from build123d import *

# Parameters (mm, degrees)
SKETCH_1_W          = 30
SKETCH_1_H          = 30
EXTRUDE_1_DEPTH     = 65
CUT_EXTRUDE_1_DEPTH = 54
CUT_EXTRUDE_2_DEPTH = 25
EXTRUDE_START       = -5.5
EXTRUDE_2_DEPTH     = 49.5
FILLET_1_R          = 0.1
SKETCH_6_R          = 3.5
CUT_EXTRUDE_3_DEPTH = 5
EXTRUDE_START_2     = 0.2
SKETCH_7_R          = 4.5
SKETCH_7_R_2        = 3.5
EXTRUDE_3_DEPTH     = 0.2
SKETCH_8_R          = 2.1
EXTRUDE_4_DEPTH     = 8
SKETCH_9_R          = 0.3
CUT_EXTRUDE_4_DEPTH = 8
CHAMFER_1_SIZE      = 1
CHAMFER_1_SIZE2     = 0.577350269
FILLET_2_R          = 0.1
FILLET_3_R          = 0.2
SKETCH_10_R         = 1.25
CUT_EXTRUDE_5_DEPTH = 5
SKETCH_11_R         = 1.25
CUT_EXTRUDE_6_DEPTH = 5
CUT_EXTRUDE_START   = -5
SKETCH_12_R         = 1.25
CUT_EXTRUDE_7_DEPTH = 5


with BuildPart() as part:
    # 草图1 → 凸台-拉伸1 (new body)
    with BuildSketch(Plane.XY):
        with Locations((0, 15)):
            Rectangle(SKETCH_1_W, SKETCH_1_H)
    extrude(amount=-EXTRUDE_1_DEPTH)

    # 草图2 → 切除-拉伸1 (cut)
    with BuildSketch(Plane(origin=(0, 0, -65), x_dir=(-1, 0, 0), z_dir=(0, 0, -1))):
        with BuildLine():
            Line((-9, 0.677124344), (-9, 0))
            Line((-9, 0), (-6, 0))
            Line((-6, 0), (-6, 0.677124344))
            ThreePointArc((-6, 0.677124344), (-5.719957697, 1.088161527), (-5.55, 1.555590279))
            Line((-5.55, 1.555590279), (-5.55, 2.8))
            Line((-5.55, 2.8), (-9.45, 2.8))
            Line((-9.45, 2.8), (-9.45, 1.555590279))
            ThreePointArc((-9.45, 1.555590279), (-9.280042303, 1.088161527), (-9, 0.677124344))
        make_face()
        with BuildLine():
            Line((5.55, 2.8), (5.55, 1.555590279))
            ThreePointArc((5.55, 1.555590279), (5.719957697, 1.088161527), (6, 0.677124344))
            Line((6, 0.677124344), (6, 0))
            Line((6, 0), (9, 0))
            Line((9, 0), (9, 0.677124344))
            ThreePointArc((9, 0.677124344), (9.280042303, 1.088161527), (9.45, 1.555590279))
            Line((9.45, 1.555590279), (9.45, 2.8))
            Line((9.45, 2.8), (5.55, 2.8))
        make_face()
    extrude(amount=-CUT_EXTRUDE_1_DEPTH, mode=Mode.SUBTRACT)

    # 草图3 → 切除-拉伸2 (cut)
    with BuildSketch(Plane(origin=(0, 0, -65), x_dir=(-1, 0, 0), z_dir=(0, 0, -1))):
        with BuildLine():
            Line((-14.322875656, 9), (-15, 9))
            Line((-15, 9), (-15, 6))
            Line((-15, 6), (-14.322875656, 6))
            ThreePointArc((-14.322875656, 6), (-13.911838473, 5.719957697), (-13.444409721, 5.55))
            Line((-13.444409721, 5.55), (-12.2, 5.55))
            Line((-12.2, 5.55), (-12.2, 9.45))
            Line((-12.2, 9.45), (-13.444409721, 9.45))
            ThreePointArc((-13.444409721, 9.45), (-13.911838473, 9.280042303), (-14.322875656, 9))
        make_face()
        with BuildLine():
            Line((-12.2, 20.55), (-13.444409721, 20.55))
            ThreePointArc((-13.444409721, 20.55), (-13.911838473, 20.719957697), (-14.322875656, 21))
            Line((-14.322875656, 21), (-15, 21))
            Line((-15, 21), (-15, 24))
            Line((-15, 24), (-14.322875656, 24))
            ThreePointArc((-14.322875656, 24), (-13.911838473, 24.280042303), (-13.444409721, 24.45))
            Line((-13.444409721, 24.45), (-12.2, 24.45))
            Line((-12.2, 24.45), (-12.2, 20.55))
        make_face()
        with BuildLine():
            Line((14.322875656, 21), (15, 21))
            Line((15, 21), (15, 24))
            Line((15, 24), (14.322875656, 24))
            ThreePointArc((14.322875656, 24), (13.911838473, 24.280042303), (13.444409721, 24.45))
            Line((13.444409721, 24.45), (12.2, 24.45))
            Line((12.2, 24.45), (12.2, 20.55))
            Line((12.2, 20.55), (13.444409721, 20.55))
            ThreePointArc((13.444409721, 20.55), (13.911838473, 20.719957697), (14.322875656, 21))
        make_face()
        with BuildLine():
            Line((12.2, 9.45), (13.444409721, 9.45))
            ThreePointArc((13.444409721, 9.45), (13.911838473, 9.280042303), (14.322875656, 9))
            Line((14.322875656, 9), (15, 9))
            Line((15, 9), (15, 6))
            Line((15, 6), (14.322875656, 6))
            ThreePointArc((14.322875656, 6), (13.911838473, 5.719957697), (13.444409721, 5.55))
            Line((13.444409721, 5.55), (12.2, 5.55))
            Line((12.2, 5.55), (12.2, 9.45))
        make_face()
    extrude(amount=-CUT_EXTRUDE_2_DEPTH, mode=Mode.SUBTRACT)

    # 草图5 → 凸台-拉伸2 (add)
    with BuildSketch(Plane(origin=(0, 0, -65), x_dir=(-1, 0, 0), z_dir=(0, 0, -1)).offset(EXTRUDE_START)):
        with BuildLine():
            Line((-1.5, 30.677124344), (-1.5, 30))
            Line((-1.5, 30), (-0.5, 30))
            Line((-0.5, 30), (-0.5, 31.07225346))
            Line((-0.5, 31.07225346), (-1.165769145, 32.5))
            Line((-1.165769145, 32.5), (-1.95, 32.5))
            Line((-1.95, 32.5), (-1.95, 31.555590279))
            ThreePointArc((-1.95, 31.555590279), (-1.780042303, 31.088161527), (-1.5, 30.677124344))
        make_face()
        with BuildLine():
            Line((1.5, 30), (1.5, 30.677124344))
            ThreePointArc((1.5, 30.677124344), (1.780042303, 31.088161527), (1.95, 31.555590279))
            Line((1.95, 31.555590279), (1.95, 32.5))
            Line((1.95, 32.5), (1.165769145, 32.5))
            Line((1.165769145, 32.5), (0.5, 31.07225346))
            Line((0.5, 31.07225346), (0.5, 30))
            Line((0.5, 30), (1.5, 30))
        make_face()
    extrude(amount=-EXTRUDE_2_DEPTH)

    # 圆角1
    fillet_1_edges = [part.edges().sort_by_distance(p)[0] for p in [
        (1.557884573, 32.5, -10),
        (1.95, 32.5, -34.75),
        (1.165769145, 32.5, -34.75),
        (1.557884573, 32.5, -59.5),
        (-1.557884573, 32.5, -10),
        (-1.165769145, 32.5, -34.75),
        (-1.95, 32.5, -34.75),
        (-1.557884573, 32.5, -59.5),
    ]]
    fillet(fillet_1_edges, radius=FILLET_1_R)

    # 草图6 → 切除-拉伸3 (cut)
    with BuildSketch(Plane.XY):
        with Locations((0, 15)):
            Circle(SKETCH_6_R)
    extrude(amount=-CUT_EXTRUDE_3_DEPTH, mode=Mode.SUBTRACT)

    # 草图7 → 凸台-拉伸3 (add)
    with BuildSketch(Plane.XY.offset(EXTRUDE_START_2)):
        with Locations(Location((0, 15, 0), (0, 0, 180))):
            Circle(SKETCH_7_R)
        with Locations((0, 15)):
            Circle(SKETCH_7_R_2, mode=Mode.SUBTRACT)
    extrude(amount=-EXTRUDE_3_DEPTH)

    # 草图8 → 凸台-拉伸4 (add)
    with BuildSketch(Plane.XY.offset(-5)):
        with Locations((0, 15)):
            Circle(SKETCH_8_R)
    extrude(amount=EXTRUDE_4_DEPTH)

    # 草图9 → 切除-拉伸4 (cut)
    with BuildSketch(Plane.XY.offset(3)):
        with Locations((0, 15)):
            Circle(SKETCH_9_R)
    extrude(amount=-CUT_EXTRUDE_4_DEPTH, mode=Mode.SUBTRACT)

    # 倒角1
    chamfer_1_edges = [part.edges().sort_by_distance(p)[0] for p in [
        (-2.1, 15, 3),
    ]]
    chamfer_1_side = [part.faces().sort_by_distance(p)[0] for p in [
        (-2.1, 15, -1),
    ]]
    chamfer(chamfer_1_edges, length=CHAMFER_1_SIZE, length2=CHAMFER_1_SIZE2, reference=chamfer_1_side[0])

    # 圆角2
    fillet_2_edges = [part.edges().sort_by_distance(p)[0] for p in [
        (-1.522649731, 15, 3),
    ]]
    fillet(fillet_2_edges, radius=FILLET_2_R)

    # 圆角3
    fillet_3_edges = [part.edges().sort_by_distance(p)[0] for p in [
        (15, 3, -65),
        (-15, 15, -65),
        (-15, 22.5, -40),
        (-15, 24, -52.5),
        (-15, 21, -52.5),
        (-15, 3, -65),
        (0, 30, -65),
        (-15, 7.5, -40),
        (-15, 9, -52.5),
        (-15, 6, -52.5),
        (12, 0, -65),
        (7.5, 0, -11),
        (6, 0, -38),
        (9, 0, -38),
        (0, 0, -65),
        (-15, 27, -65),
        (-7.5, 0, -11),
        (-9, 0, -38),
        (-6, 0, -38),
        (0, 30, 0),
        (15, 15, 0),
        (0, 0, 0),
        (-15, 15, 0),
        (15, 15, -65),
        (-12, 0, -65),
        (15, 7.5, -40),
        (15, 6, -52.5),
        (15, 9, -52.5),
        (-15, 30, -32.5),
        (15, 30, -32.5),
        (15, 0, -32.5),
        (-15, 0, -32.5),
        (15, 27, -65),
        (15, 22.5, -40),
        (15, 21, -52.5),
        (15, 24, -52.5),
    ]]
    fillet(fillet_3_edges, radius=FILLET_3_R)

    # 草图10 → 切除-拉伸5 (cut)
    with BuildSketch(Plane.XY):
        with Locations((-12.25, 3.75)):
            Circle(SKETCH_10_R)
        with Locations((12.25, 3.75)):
            Circle(SKETCH_10_R)
    extrude(amount=-CUT_EXTRUDE_5_DEPTH, mode=Mode.SUBTRACT)

    # 草图11 → 切除-拉伸6 (cut)
    with BuildSketch(Plane(origin=(15, 0, 0), x_dir=(0, 0, -1), z_dir=(1, 0, 0))):
        with Locations((3.75, 3.75)):
            Circle(SKETCH_11_R)
    extrude(amount=-CUT_EXTRUDE_6_DEPTH, mode=Mode.SUBTRACT)

    # 草图12 → 切除-拉伸7 (cut)
    with BuildSketch(Plane.ZY.offset(15).offset(CUT_EXTRUDE_START)):
        with Locations(Location((-3.75, 3.75, 0), (0, 0, 180))):
            Circle(SKETCH_12_R)
    extrude(amount=CUT_EXTRUDE_7_DEPTH, mode=Mode.SUBTRACT)


solid = part.part
For this review, take the finished solid that the model builds, in its own axes (mm). A direction names the side the tool comes from. Coordinates: 2 decimals unless noted, no trailing zeros. Answer as CSV lines item,"result". Start each with the question number.
1) To check wall thickness, follow line 1 along Z through (x, y) = (-10.6, 3.75); line 2 along X through (y, z) = (3.75, -2); line 3 along Y through (x, z) = (11.35, -3.75). State the ranges of each line that lie inside material, in increasing order. Write a range as [from, to].
2) Draft analysis for pull direction X (two halves, no side actions). For faces 1 (the flat face through (1, 31, -10)), 2 (the flat face through (-5.55, 2, -38)), state which applies: +X half, -X half, draft (parallel to the pull), parting line (faces both ways), or undercut.
3) Insertion check: P1, Ø10, axis at x = -5, z = -42, coming from the +Y side; P2, Ø0.8, axis at x = 6.5, y = 1.5, coming from the -Z side; P3, Ø6, axis at x = -11.5, z = -30.5, coming from the +Y side; P4, Ø0.8, axis at y = 3.5, z = -4, coming from the +X side. Each pin has a flat end and moves straight along its axis. Give the tip position at first contact, or say it passes through.
4) Machinability: for faces 3 (the flat face through (-13, 24.45, -53)), 4 (the cylindrical face through (-13.9, 3.7, -2.5)), 5 (the cylindrical face through (-12.2, 5, -4.6)), which of the approach directions +Z, -Z, +X, -X, +Y, -Y give a long, thin tool a straight path to every point of the face, cutting with its end or side? Answer none if there is none.
Result:
1,line 1,"[-65, -5], [-2.5, 0]"
1,line 2,"[-15, -13.5], [-11, 11], [13.5, 15]"
1,line 3,"[0, 2.5], [5, 30]"
2,face 1,"draft"
2,face 2,"undercut"
3,P1,"y = 32.5"
3,P2,"z = -11"
3,P3,"y = 30"
3,P4,"x = 10"
4,face 3,"-Z"
4,face 4,"-X"
4,face 5,"+Z"
